Geometry: see drawing. Coordinates: mm, zero at the bounding-box minimum. Give positions to 0.01 mm unless a question says otherwise; leave off trailing zeros. Write each loop counter-clockwise with the first axis right and the second up, starting at its lowest first coordinate (ties: lowest second). Pieces come first, ordered by that corner, then holes. Notation, with made-up numbers: (-34.5, 73) - (-19.5, 73) arc R27 cw to (-19.5, 91) - close; hole circle Ø6 at (33.5, -28.75). An arc over 180 degrees is marked (long way). Use a Markdown table: item, result. Add a question column.
1. Pin query (flat end, axial travel): pin 1 (2.5 mm diameter, centred on x = 4.5, y = 5, fed in from +Z); pin 2 (5.5 mm diameter, centred on x = 156, y = 154, fed in from +Z). Return the tip coordinate at first contact, or that it passes through.
2. Section query A-A, the plane y = 141. Return loops of the section in (x, z).
3. Section query C-C, the plane z = 7.75. Return loops of the section in (x, y), plus the area to 3 significant figures.
4. Section query D-D, the plane x = 5. Return loops of the section in (y, z).
5. Material intervals for probe 1 along X at (y, z) = (155, 7.1); probe 2 along X at (y, z) = (51.5, 8), sorted ascending.
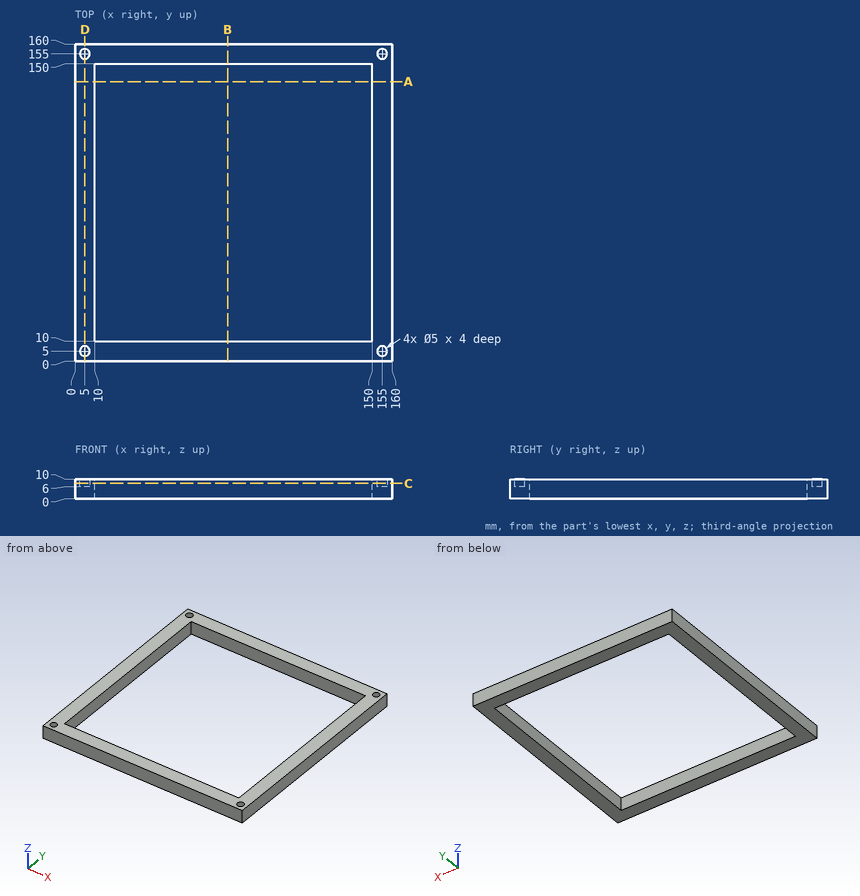
Result sheet:
| question | item | result |
|---|---|---|
| 1 | pin 1 | stops at z = 6 |
| 1 | pin 2 | stops at z = 10 |
| 2 | outline | (0, 0) - (10, 0) - (10, 10) - (0, 10) - close; (150, 0) - (160, 0) - (160, 10) - (150, 10) - close |
| 3 | outline | (0, 0) - (160, 0) - (160, 160) - (0, 160) - close; hole circle Ø5 at (5, 5); hole circle Ø5 at (5, 155); hole (10, 10) - (150, 10) - (150, 150) - (10, 150) - close; hole circle Ø5 at (155, 5); hole circle Ø5 at (155, 155) |
| 3 | area | 5,920 mm² |
| 4 | outline | (0, 0) - (160, 0) - (160, 10) - (157.5, 10) - (157.5, 6) - (152.5, 6) - (152.5, 10) - (7.5, 10) - (7.5, 6) - (2.5, 6) - (2.5, 10) - (0, 10) - close |
| 5 | probe 1 | x = 0 to 2.5, 7.5 to 152.5, 157.5 to 160 |
| 5 | probe 2 | x = 0 to 10, 150 to 160 |
